The listing builds one solid part. Answer for the finished solid, in the listing's coordinates (mm). A direction names the side the tool comes from. Give positions to 0.01 mm unless a question says otherwise; leave off trailing zeros. Loops run counter-clockwise (first coordinate to the right, second up) from the corner with the lowest first, then second, coordinate; pieces in that order, holes last. Notation, with made-up numbers: (-8, 80.25) - (47, 80.25) arc R26 ccw to (47, 118.25) - close; hole circle Ø1 at (67.5, 63). An arc over 180 degrees is marked (long way). Write each question's results on one line, items separated by ' | '.
from build123d import *

# Parameters (mm, degrees)
F0_R     = 12.7
F1_DEPTH = 25.4
F3_DEPTH = 76.2
F4_R     = 12.7
F5_DEPTH = 25.4


with BuildPart() as f1:
    # F0 (on Top) → F1 (new body)
    with BuildSketch(Plane.XY):
        Polygon((2.805811, 78.11977), (-73.394189, 78.11977), (-73.394189, 27.31977), (-98.794189, 27.31977), (-98.794189, -48.88023), (-73.394189, -48.88023), (-22.594189, -48.88023), (-22.594189, -99.68023), (2.805811, -99.68023), (2.805811, -48.88023), align=None)
        with Locations((-35.294189, 40.01977)):
            Circle(F0_R, mode=Mode.SUBTRACT)
    extrude(amount=F1_DEPTH)

    # F2 (on face) → F3 (join)
    with BuildSketch(Plane.XY.offset(25.4)):
        Polygon((2.805811, -23.48023), (-98.794189, -23.48023), (-98.794189, -48.88023), (-22.594189, -48.88023), (-22.594189, -99.68023), (2.805811, -99.68023), align=None)
    extrude(amount=F3_DEPTH)

    # F4 (on face) → F5 (cut)
    with BuildSketch(Plane.XZ.offset(48.88023)):
        with Locations((-59.483197, 63.5)):
            Circle(F4_R)
    extrude(amount=-F5_DEPTH, mode=Mode.SUBTRACT)


solid = f1.part
Item 1: Flat-ended cylindrical pins translate along their axes: P1, Ø1.5, axis at x = -33, z = 64.5, coming from the -Y side; P2, Ø2, axis at x = -55.5, y = -4.5, coming from the +Z side; P3, Ø5, axis at x = -76, z = 66, coming from the +Y side. Find the tip coordinate at first contact, or state that the pin passes through.
Values found:
P1: stops at y = -48.88 | P2: stops at z = 25.4 | P3: stops at y = -23.48
Item 2: A cutting plane is placed at B-B, the plane y = -25.5. Determine the outline of the cut face in (x, z), plus the area to 3 significant figures.
Values found:
outline: (-98.79, 0) - (2.81, 0) - (2.81, 101.6) - (-98.79, 101.6) - close; hole circle Ø25.4 at (-59.48, 63.5) | area: 9,820 mm²
Item 3: A cutting plane is placed at D-D, the plane x = -15. Determine the outline of the cut face in (y, z).
Values found:
outline: (-99.68, 0) - (78.12, 0) - (78.12, 25.4) - (-23.48, 25.4) - (-23.48, 101.6) - (-99.68, 101.6) - close
Item 4: For a pull along Z with two mould halves and no side action, classify faces 4 (the face through (-22.594, -74, 50)), 5 (the face through (-68.844, -36.358, 72.083)), 6 (the face through (-37, 10, 0)), 7 (the face through (-49, 28, 25.4)) as released by +Z, released by -Z, zero draft, split by the parting line, or undercut.
Values found:
face 4: zero draft | face 5: undercut | face 6: released by -Z | face 7: released by +Z
Item 5: A cutting plane is placed at A-A, the plane z = 63.5. Determine the outline of the cut face in (x, y).
Values found:
outline: (-98.79, -48.88) - (-72.18, -48.88) - (-72.18, -23.48) - (-98.79, -23.48) - close; (-46.78, -48.88) - (-22.59, -48.88) - (-22.59, -99.68) - (2.81, -99.68) - (2.81, -23.48) - (-46.78, -23.48) - close
Item 6: Find the intervals of material crossed by line 1 along X through (y, z) = (-43, 63); line 2 along X through (y, z) = (-72, 85); line 3 along Z through (x, y) = (-76, 15), in increasing order. Write a range as [from, to].
Values found:
line 1: x = [-98.79, -72.17], [-46.79, 2.81] | line 2: x = [-22.59, 2.81] | line 3: z = [0, 25.4]
Item 7: A cutting plane is placed at C-C, the plane x = -68.5. Determine the outline of the cut face in (y, z), plus the area to 3 significant figures.
Values found:
outline: (-48.88, 0) - (78.12, 0) - (78.12, 25.4) - (-23.48, 25.4) - (-23.48, 54.56) - (-48.88, 54.56) - close; (-48.88, 72.44) - (-23.48, 72.44) - (-23.48, 101.6) - (-48.88, 101.6) - close | area: 4,710 mm²
Item 8: For faces 1 (the face through (-73.394, 53, 13)), 2 (the face through (-61, -48.88, 50)), 3 (the face through (-47, -23.48, 54)), determine the directions among +Z, -Z, +X, -X, +Y, -Y from which every point of the face is accessible in a straight line to the end or side of a thin tool.
Values found:
face 1: +Z, -Z, -X, +Y | face 2: +Z, -Z, -X, -Y | face 3: +Z, +X, -X, +Y
